Geometry: final body of the model. Coordinates: model frame, mm. Face numbers are marked on the shaded views. Coordinates: 2 decimals unless noted, no trailing zeros. Order: outer loops, then holes, each group sorted by start corner. A loop starts at its lowest first (then second) coordinate and runs counter-clockwise, first axis right, second up. Notation, with made-up numbers: M 53.25,86 L 97.25,86 A21 cw 97.25,101 Z; hole C 44.25,64.5 d6. An arc over 180 degrees is marked long. Write item = value, one per line. Start each with the question number.
```python
from build123d import *

# Parameters (mm, degrees)
F0_R     = 2.8
F1_DEPTH = 12
F0_W     = 6.25
F0_H     = 9.5
F0_R_2   = 1.4
F2_DEPTH = 17
F3_SIZE  = 2.2
F4_START = 8
F0_R_3   = 1.575
F4_DEPTH = 3
F5_W     = 68.25
F5_H     = 47.75
F5_W_2   = 8.775
F5_H_2   = 36.234842279
F5_W_3   = 54.475
F5_H_3   = 24.4
F6_DEPTH = 28
F7_SIZE  = 2


# Not quite as in the source:
# - a feature names something its author has since deleted; it is built from what else it names


with BuildPart() as f1:
    # F0 (on Front) → F1 (new body)
    with BuildSketch(Plane.XZ):
        Polygon((-36.875, -54.75), (36.875, -54.75), (36.875, -45.25), (43.125, -45.25), (43.125, 45.25), (36.875, 45.25), (36.875, 54.75), (-36.875, 54.75), (-36.875, 45.25), (-43.125, 45.25), (-43.125, -45.25), (-36.875, -45.25), align=None)
        with Locations((-31, -49.75)):
            Circle(F0_R, mode=Mode.SUBTRACT)
        with Locations((30.8, -49.75)):
            Circle(F0_R, mode=Mode.SUBTRACT)
        with Locations((16.55, -11.55)):
            Circle(F0_R, mode=Mode.SUBTRACT)
    extrude(amount=F1_DEPTH)

    # F0 (on Front) → F2 (join)
    with BuildSketch(Plane.XZ):
        with Locations((40, -50)):
            Rectangle(F0_W, F0_H)
        Polygon((40, -46.4492958445), (43.075, -48.2246479222), (43.075, -51.7753520778), (40, -53.5507041555), (36.925, -51.7753520778), (36.925, -48.2246479222), align=None, mode=Mode.SUBTRACT)
        with Locations((-40, -50)):
            Rectangle(F0_W, F0_H)
        Polygon((-40, -46.4492958445), (-36.925, -48.2246479222), (-36.925, -51.7753520778), (-40, -53.5507041555), (-43.075, -51.7753520778), (-43.075, -48.2246479222), align=None, mode=Mode.SUBTRACT)
        with Locations((-40, 50)):
            Rectangle(F0_W, F0_H)
        Polygon((-40, 53.5507041555), (-36.925, 51.7753520778), (-36.925, 48.2246479222), (-40, 46.4492958445), (-43.075, 48.2246479222), (-43.075, 51.7753520778), align=None, mode=Mode.SUBTRACT)
        with Locations((40, 50)):
            Rectangle(F0_W, F0_H)
        Polygon((40, 46.4492958445), (36.925, 48.2246479222), (36.925, 51.7753520778), (40, 53.5507041555), (43.075, 51.7753520778), (43.075, 48.2246479222), align=None, mode=Mode.SUBTRACT)
        Polygon((-36.925, -51.7753520778), (-36.925, -48.2246479222), (-40, -46.4492958445), (-43.075, -48.2246479222), (-43.075, -51.7753520778), (-40, -53.5507041555), align=None)
        with Locations((-40, -50)):
            Circle(F0_R_2, mode=Mode.SUBTRACT)
        Polygon((43.075, -51.7753520778), (43.075, -48.2246479222), (40, -46.4492958445), (36.925, -48.2246479222), (36.925, -51.7753520778), (40, -53.5507041555), align=None)
        with Locations((40, -50)):
            Circle(F0_R_2, mode=Mode.SUBTRACT)
        Polygon((36.925, 51.7753520778), (36.925, 48.2246479222), (40, 46.4492958445), (43.075, 48.2246479222), (43.075, 51.7753520778), (40, 53.5507041555), align=None)
        with Locations((40, 50)):
            Circle(F0_R_2, mode=Mode.SUBTRACT)
        Polygon((-36.925, 48.2246479222), (-36.925, 51.7753520778), (-40, 53.5507041555), (-43.075, 51.7753520778), (-43.075, 48.2246479222), (-40, 46.4492958445), align=None)
        with Locations((-40, 50)):
            Circle(F0_R_2, mode=Mode.SUBTRACT)
    extrude(amount=F2_DEPTH)

    # F3
    f3_edges = [f1.edges().sort_by_distance(p)[0] for p in [
        (-40, -17, -45.25),
        (-40, -17, -54.75),
        (40, -17, -45.25),
        (40, -17, -54.75),
        (-40, -17, 54.75),
        (-40, -17, 45.25),
        (40, -17, 54.75),
        (40, -17, 45.25),
    ]]
    chamfer(f3_edges, length=F3_SIZE)

    # F0 (on Front) → F4 (join)
    with BuildSketch(Plane.XZ.offset(F4_START)):
        with Locations((16.55, -11.55)):
            Circle(F0_R)
        with Locations((16.55, -11.55)):
            Circle(F0_R_3, mode=Mode.SUBTRACT)
        with Locations((30.8, -49.75)):
            Circle(F0_R)
        with Locations((30.8, -49.75)):
            Circle(F0_R_3, mode=Mode.SUBTRACT)
        with Locations((-31, -49.75)):
            Circle(F0_R)
        with Locations((-31, -49.75)):
            Circle(F0_R_3, mode=Mode.SUBTRACT)
    extrude(amount=F4_DEPTH)

    # F5 (on face) → F6 (cut)
    with BuildSketch(Plane(origin=(0, 0, 0), x_dir=(-1, 0, 0), z_dir=(0, 1, 0))):
        with Locations((0, 21.875)):
            Rectangle(F5_W, F5_H)
        with Locations((-29.7375, -25.6325788605)):
            Rectangle(F5_W_2, F5_H_2)
        with Locations((6.8875, -31.55)):
            Rectangle(F5_W_3, F5_H_3)
    extrude(amount=-F6_DEPTH, mode=Mode.SUBTRACT)

    # F7
    f7_edges = [f1.edges().sort_by_distance(p)[0] for p in [
        (0, -12, -2),
        (-34.125, -12, 21.875),
        (0, -12, 45.75),
        (34.125, -12, 21.875),
        (34.125, -12, -25.632579),
        (29.7375, -12, -7.515158),
        (25.35, -12, -25.632579),
        (29.7375, -12, -43.75),
        (-6.8875, -12, -43.75),
        (20.35, -12, -31.55),
        (-6.8875, -12, -19.35),
        (-34.125, -12, -31.55),
    ]]
    chamfer(f7_edges, length=F7_SIZE)


solid = f1.part
```
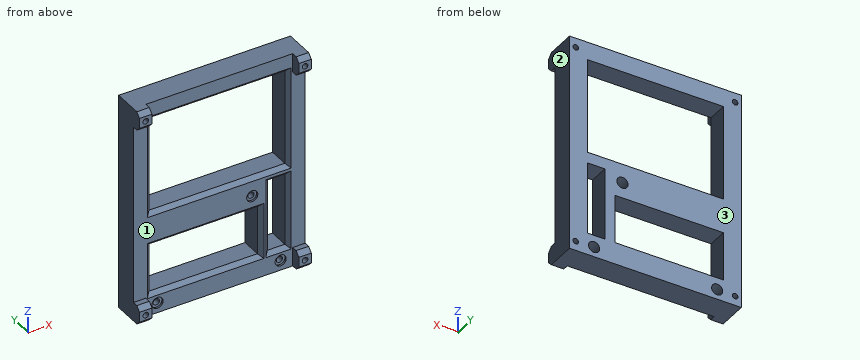
Item 1: First-contact query: pin 1 (4.5 mm diameter, centred on x = -30.5, z = -49, fed in from +Y); pin 2 (6 mm diameter, centred on x = -15, z = -15, fed in from -Y); pin 3 (2.5 mm diameter, centred on x = -31, z = -49.75, fed in from -Y); pin 4 (1.7 mm diameter, centred on x = 32, z = -51, fed in from -Y). Flat tips, straight axial feed; report the tip coordinate or a pass-through.
Item 2: Section query B-B on x = 30.8. Output: boundary loops of the cut face in (y, z) (3 decimals), and give its area (3 significant figures).
Item 3: Section query A-A on z = -11.55. Output: boundary loops of the cut face in (x, y) (3 decimals), and give its area (3 significant figures).
Item 4: Material intervals for probe 1 along Z at (x, y) = (7, -8); probe 2 along Z at (x, y) = (-31, -9.05) (3 decimals); probe 3 along Z at (x, y) = (-31, -10.25) (3 decimals), sorted ascending. Write a range as [from, to].
Item 5: Draft query along X for the marked faces 1, 2 and 3. Return one class per face: pulls with the +X half, pulls with the -X half, needs draft (parallel to the pull), parting line crosses it, or undercut.
Item 6: Section query C-C on x = -40. Output: boundary loops of the cut face in (y, z), and give its area (3 significant figures).
Item 7: Section query D-D on z = 17. Output: boundary loops of the cut face in (x, y) (3 decimals).
Ans:
q1.pin_1 = 0
q1.pin_2 = -12
q1.pin_3 = through
q1.pin_4 = -11
q2.outline = M -12,-54.75 L 0,-54.75 L 0,-52.55 L -8,-52.55 L -8,-51.325 L -11,-51.325 L -11,-52.55 L -12,-52.55 Z; M -12,-46.95 L -11,-46.95 L -11,-48.175 L -8,-48.175 L -8,-46.95 L 0,-46.95 L 0,-43.75 L -10,-43.75 L -12,-45.75 Z; M -12,-5.515 L -10,-7.515 L 0,-7.515 L 0,-2 L -10,-2 L -12,-4 Z; M -12,47.75 L -10,45.75 L 0,45.75 L 0,54.75 L -12,54.75 Z
q2.area = 238 mm^2
q3.outline = M -43.125,-12 L 13.75,-12 L 13.75,-11 L 14.975,-11 L 14.975,-8 L 13.75,-8 L 13.75,0 L -43.125,0 Z; M 18.125,-11 L 19.35,-11 L 19.35,-12 L 23.35,-12 L 25.35,-10 L 25.35,0 L 19.35,0 L 19.35,-8 L 18.125,-8 Z; M 34.125,-10 L 36.125,-12 L 43.125,-12 L 43.125,0 L 34.125,0 Z
q3.area = 866 mm^2
q4.probe_1 = [-54.75, -43.75], [-19.35, -2], [45.75, 54.75]
q4.probe_2 = [-54.75, -51.325], [-48.175, -43.75], [-19.35, -2], [45.75, 54.75]
q4.probe_3 = [-54.75, -51.325], [-48.175, -44], [-19.1, -2.25], [46, 54.75]
q5.face_1 = undercut
q5.face_2 = pulls with the +X half
q5.face_3 = needs draft
q6.outline = M -17,-52.55 L -14.8,-54.75 L 0,-54.75 L 0,-51.4 L -17,-51.4 Z; M -17,-48.6 L 0,-48.6 L 0,48.6 L -17,48.6 L -17,47.45 L -14.8,45.25 L -12,45.25 L -12,-45.25 L -14.8,-45.25 L -17,-47.45 Z; M -17,51.4 L 0,51.4 L 0,54.75 L -14.8,54.75 L -17,52.55 Z
q6.area = 1,300 mm^2
q7.outline = M -43.125,-12 L -36.125,-12 L -34.125,-10 L -34.125,0 L -43.125,0 Z; M 34.125,-10 L 36.125,-12 L 43.125,-12 L 43.125,0 L 34.125,0 Z
